```python
from build123d import *

# Parameters (mm, degrees)
SKETCH1_R           = 4.5
BOSS_EXTRUDE1_DEPTH = 6
SKETCH2_R           = 1.6
SKETCH2_R_2         = 0.7
BOSS_EXTRUDE2_DEPTH = 1.6
SKETCH3_R           = 0.7
BOSS_EXTRUDE3_DEPTH = 0.8
BOSS_EXTRUDE4_START = -4
SKETCH4_R           = 0.6
BOSS_EXTRUDE4_DEPTH = 3
CUT_EXTRUDE1_START  = -2
CUT_EXTRUDE1_DEPTH  = 1
CUT_EXTRUDE2_START  = -4
CUT_EXTRUDE2_DEPTH  = 1
FILLET1_R           = 0.3
SKETCH5_R           = 2.2
CUT_EXTRUDE4_DEPTH  = 19.08212732
SKETCH9_R           = 3.2
SKETCH9_R_2         = 2.2
CUT_EXTRUDE5_DEPTH  = 2


with BuildPart() as part:
    # Sketch1 → Boss-Extrude1 (new body)
    with BuildSketch(Plane(origin=(0, 0, 0), x_dir=(1, 0, 0), z_dir=(0, 1, 0))):
        with Locations(Location((0, 0, 0), (0, 0, 270))):
            Circle(SKETCH1_R)
    extrude(amount=BOSS_EXTRUDE1_DEPTH)

    # Sketch2 → Boss-Extrude2 (add)
    # profile 1 of 4: a face of its own
    with BuildSketch(Plane.XZ):
        with BuildLine():
            ThreePointArc((-0.717333438, -4.442457961), (-2.25, -3.897114317), (-3.488614731, -2.842457961))
            Line((-3.488614731, -2.842457961), (-4.635640646, -4.829165125))
            ThreePointArc((-4.635640646, -4.829165125), (-2.835889528, -4.083683803), (-1.65, -5.629165125))
            ThreePointArc((-1.65, -5.629165125), (-1.704518678, -6.043275597), (-1.864359354, -6.429165125))
            Line((-1.864359354, -6.429165125), (-0.717333438, -4.442457961))
        make_face()
    # profile 2 of 4: a face of its own
    with BuildSketch(Plane.XZ):
        with Locations((-3.25, -5.629165125)):
            Circle(SKETCH2_R)
        with Locations(Location((-3.25, -5.629165125, 0), (0, 0, 270))):
            Circle(SKETCH2_R_2, mode=Mode.SUBTRACT)
    # profile 3 of 4: a face of its own
    with BuildSketch(Plane.XZ):
        with Locations((-3.25, 5.629165125)):
            Circle(SKETCH2_R)
        with Locations(Location((-3.25, 5.629165125, 0), (0, 0, 270))):
            Circle(SKETCH2_R_2, mode=Mode.SUBTRACT)
    # profile 4 of 4: a face of its own
    with BuildSketch(Plane.XZ):
        with BuildLine():
            ThreePointArc((-1.65, 5.629165125), (-2.835889528, 4.083683803), (-4.635640646, 4.829165125))
            Line((-4.635640646, 4.829165125), (-3.488614731, 2.842457961))
            ThreePointArc((-3.488614731, 2.842457961), (-2.25, 3.897114317), (-0.717333438, 4.442457961))
            Line((-0.717333438, 4.442457961), (-1.864359354, 6.429165125))
            ThreePointArc((-1.864359354, 6.429165125), (-1.704518678, 6.043275597), (-1.65, 5.629165125))
        make_face()
    extrude(amount=-BOSS_EXTRUDE2_DEPTH)

    # Sketch3 → Boss-Extrude3 (add, symmetric)
    with BuildSketch(Plane.XY):
        with BuildLine():
            Line((-3.5, 6), (-6.5, 6))
            ThreePointArc((-6.5, 6), (-8.1, 4.4), (-6.5, 2.8))
            Line((-6.5, 2.8), (-3.5, 2.8))
            Line((-3.5, 2.8), (-3.5, 6))
        make_face()
        with Locations((-6.5, 4.4)):
            Circle(SKETCH3_R, mode=Mode.SUBTRACT)
    extrude(amount=BOSS_EXTRUDE3_DEPTH, both=True)

    # Sketch4 → Boss-Extrude4 (add)
    with BuildSketch(Plane(origin=(0, 6, 0), x_dir=(1, 0, 0), z_dir=(0, 1, 0)).offset(BOSS_EXTRUDE4_START)):
        with BuildLine():
            ThreePointArc((1.029929577, 4.380553055), (4.5, 0), (1.029929577, -4.380553055))
            Line((1.029929577, -4.380553055), (14.486091549, -1.216820293))
            ThreePointArc((14.486091549, -1.216820293), (15.45, 0), (14.486091549, 1.216820293))
            Line((14.486091549, 1.216820293), (1.029929577, 4.380553055))
        make_face()
        with BuildLine():
            ThreePointArc((4.931081365, -2.436069903), (5.5, 0), (4.931081365, 2.436069903))
            Line((4.931081365, 2.436069903), (12.080503997, 0.75514018))
            ThreePointArc((12.080503997, 0.75514018), (11.982866038, 0.38316706), (11.95, 0))
            ThreePointArc((11.95, 0), (11.982866038, -0.38316706), (12.080503997, -0.75514018))
            Line((12.080503997, -0.75514018), (4.931081365, -2.436069903))
        make_face(mode=Mode.SUBTRACT)
        with Locations(Location((14.2, 0, 0), (0, 0, 270))):
            Circle(SKETCH4_R, mode=Mode.SUBTRACT)
    extrude(amount=BOSS_EXTRUDE4_DEPTH)

    # Sketch4_3 → Cut-Extrude1 (cut)
    with BuildSketch(Plane(origin=(0, 6, 0), x_dir=(1, 0, 0), z_dir=(0, 1, 0)).offset(CUT_EXTRUDE1_START)):
        with BuildLine():
            Line((12.664921694, 1.645002916), (4.108268481, 3.656792323))
            ThreePointArc((4.108268481, 3.656792323), (4.560701943, 3.074084869), (4.931081365, 2.436069903))
            Line((4.931081365, 2.436069903), (12.080503997, 0.75514018))
            ThreePointArc((12.080503997, 0.75514018), (12.319323987, 1.235134702), (12.664921694, 1.645002916))
        make_face()
    extrude(amount=CUT_EXTRUDE1_DEPTH, mode=Mode.SUBTRACT)

    # Sketch4_4 → Cut-Extrude2 (cut)
    with BuildSketch(Plane(origin=(0, 6, 0), x_dir=(1, 0, 0), z_dir=(0, 1, 0)).offset(CUT_EXTRUDE2_START)):
        with BuildLine():
            Line((12.664921694, 1.645002916), (4.108268481, 3.656792323))
            ThreePointArc((4.108268481, 3.656792323), (4.560701943, 3.074084869), (4.931081365, 2.436069903))
            Line((4.931081365, 2.436069903), (12.080503997, 0.75514018))
            ThreePointArc((12.080503997, 0.75514018), (12.319323987, 1.235134702), (12.664921694, 1.645002916))
        make_face()
    extrude(amount=CUT_EXTRUDE2_DEPTH, mode=Mode.SUBTRACT)

    # Fillet1
    fillet1_edges = [part.edges().sort_by_distance(p)[0] for p in [
        (4.931081365, 3.5, 2.436069903),
        (12.080503997, 3.5, 0.75514018),
        (12.080503997, 3.5, -0.75514018),
        (4.931081365, 3.5, -2.436069903),
    ]]
    fillet(fillet1_edges, radius=FILLET1_R)

    # Sketch5 → Cut-Extrude4 (cut, through all)
    with BuildSketch(Plane(origin=(0, 6, 0), x_dir=(1, 0, 0), z_dir=(0, 1, 0))):
        with Locations(Location((0, 0, 0), (0, 0, 270))):
            Circle(SKETCH5_R)
    extrude(amount=-CUT_EXTRUDE4_DEPTH, mode=Mode.SUBTRACT)

    # Sketch9 → Cut-Extrude5 (cut)
    with BuildSketch(Plane(origin=(0, 6, 0), x_dir=(1, 0, 0), z_dir=(0, 1, 0))):
        with Locations(Location((0, 0, 0), (0, 0, 270))):
            Circle(SKETCH9_R)
        with Locations(Location((0, 0, 0), (0, 0, 270))):
            Circle(SKETCH9_R_2, mode=Mode.SUBTRACT)
    extrude(amount=-CUT_EXTRUDE5_DEPTH, mode=Mode.SUBTRACT)


solid = part.part
```
The model under review builds one solid part; all positions refer to its coordinate system, in mm. A direction names the side the tool comes from. Coordinates: 2 decimals unless noted, no trailing zeros. Loops run counter-clockwise (first coordinate to the right, second up) from the corner with the lowest first, then second, coordinate; pieces in that order, holes last. Notation, with made-up numbers: (58, 71.25) -> (113, 71.25) arc R27 cw to (113, 103.25) -> close; hole circle Ø1 at (23, 80.25). An arc over 180 degrees is marked (long way). Answer as CSV lines item,"result".
Item 1: Take a section at A-A, the plane y = 0.9. State the section outline as (x, z) points, and give its area (3 significant figures).
Results below:
outline,"(-4.64, -4.83) arc R1.6 ccw to (-1.86, -6.43) -> (-0.72, -4.44) arc R4.5 ccw (long way) to (-0.72, 4.44) -> (-1.86, 6.43) arc R1.6 ccw to (-4.64, 4.83) -> (-3.49, 2.84) arc R4.5 ccw to (-3.49, -2.84) -> close; hole circle Ø1.4 at (-3.25, -5.63); hole circle Ø1.4 at (-3.25, 5.63); hole circle Ø4.4 at (0, 0)"
area,"66.8 mm2"
Item 2: For L1, parallel to Y at x = -6.5, z = -0.3; L2, parallel to X at y = 2.45, z = 0.75; L3, parallel to Y at x = 12.25, z = 1.25, list the stretches that pass through material, from the lowest coordinate up.
Results below:
L1,"y = 2.8 to 3.7, 5.1 to 6"
L2,"x = -4.44 to -2.07, 2.07 to 5.45, 11.92 to 15.2"
L3,"y = 2 to 5"
Item 3: Take a section at D-D, the plane x = 14.2. State the section outline as (y, z) points.
Results below:
outline,"(2, -1.28) -> (5, -1.28) -> (5, -0.6) -> (2, -0.6) -> close; (2, 0.6) -> (5, 0.6) -> (5, 1.28) -> (2, 1.28) -> close"
Item 4: Take a section at B-B, the plane y = 4.4. Count the separate pieces of the cut face and the enclosed holes in it, and give its area (3 significant figures).
Results below:
separate pieces,"2"
enclosed holes,"2"
area,"59.6 mm2"
Item 5: Draft analysis for pull direction Z (two halves, no side actions). For faces 1 (the cylindrical face through (13.67, 3.48, 0.28)), 2 (the flat face through (9, 2, 2)), 3 (the flat face through (7.852, 3.479, -2.777)), state which applies: +Z half, -Z half, draft (parallel to the pull), parting line (faces both ways), or undercut.
Results below:
face 1,"undercut"
face 2,"draft"
face 3,"-Z half"
Item 6: Insertion check: pin 1 (3 mm diameter, centred on x = -1.5, z = -0.5, fed in from +Y); pin 2 (0.8 mm diameter, centred on x = -6.5, y = 4.4, fed in from -Z) (1 decimal); pin 3 (4.5 mm diameter, centred on x = 9.5, z = 1, fed in from +Y); pin 4 (1 mm diameter, centred on x = -5.5, y = 4, fed in from -Z). Each pin has a flat end and moves straight along its axis. Give the tip position at first contact, or say it passes through.
Results below:
pin 1,"stops at y = 4"
pin 2,"passes through"
pin 3,"stops at y = 5"
pin 4,"stops at z = -0.8"
Item 7: Machinability: for faces 4 (the flat face through (-4.07, 0.79, 3.85)), 5 (the flat face through (9, 5, 2)), 6 (the cylindrical face through (-1.947, 5.014, -2.539)), 7 (the flat face through (8, 4, -2)), which of the approach directions +Z, -Z, +X, -X, +Y, -Y give a long, thin tool a straight path to every point of the face, cutting with its end or side? Answer none if there is none.
Results below:
face 4,"-X, +Y, -Y"
face 5,"+X, +Y"
face 6,"+Y"
face 7,"-Z, +Y"
Item 8: Take a section at C-C, the plane z = -5.75. State the section outline as (x, y) points.
Results below:
outline,"(-4.85, 0) -> (-3.94, 0) -> (-3.94, 1.6) -> (-4.85, 1.6) -> close; (-2.56, 0) -> (-1.47, 0) -> (-1.47, 1.6) -> (-2.56, 1.6) -> close"
